from build123d import *

# Parameters (mm, degrees)
SKETCH1_R           = 8.25
SKETCH1_R_2         = 4.25
SKETCH1_R_3         = 15.25
SKETCH1_R_4         = 11.25
SKETCH1_R_5         = 6.25
BOSS_EXTRUDE2_DEPTH = 10
SKETCH1_5_R         = 11.25
CUT_EXTRUDE5_DEPTH  = 7


with BuildPart() as part:
    # Sketch1 → Boss-Extrude2 (new body)
    # profile 1 of 7: a face of its own
    with BuildSketch(Plane.XY):
        with BuildLine():
            Line((64.758616135, -27.860720154), (22.059293714, -16.720850027))
            ThreePointArc((22.059293714, -16.720850027), (26.505216378, -19.659807339), (28.226652646, -24.703650675))
            ThreePointArc((28.226652646, -24.703650675), (20.56881743, -32.932371163), (11.81166092, -25.884925461))
            Line((11.81166092, -25.884925461), (21.633984529, -93.776995906))
            ThreePointArc((21.633984529, -93.776995906), (35.63224039, -76.382762218), (51.976848021, -91.593427362))
            ThreePointArc((51.976848021, -91.593427362), (47.525288564, -102.361722577), (36.769479911, -106.843367773))
            Line((36.769479911, -106.843367773), (86.769284535, -106.703591085))
            ThreePointArc((86.769284535, -106.703591085), (73.507639588, -83.849691589), (99.930570224, -83.823509091))
            Line((99.930570224, -83.823509091), (69.819078019, -31.715739289))
            ThreePointArc((69.819078019, -31.715739289), (70.644447296, -33.706712359), (70.925975067, -35.843520802))
            ThreePointArc((70.925975067, -35.843520802), (56.147411334, -40.887364137), (64.758616135, -27.860720154))
        make_face()
    # profile 2 of 7: a face of its own
    with BuildSketch(Plane.XY):
        with Locations((62.675975067, -35.843520802)):
            Circle(SKETCH1_R)
        with Locations((62.675975067, -35.843520802)):
            Circle(SKETCH1_R_2, mode=Mode.SUBTRACT)
    # profile 3 of 7: a face of its own
    with BuildSketch(Plane.XY):
        with Locations((36.726848021, -91.593427362)):
            Circle(SKETCH1_R_3)
        with Locations((36.726848021, -91.593427362)):
            Circle(SKETCH1_R_4, mode=Mode.SUBTRACT)
    # profile 4 of 7: a face of its own
    with BuildSketch(Plane.XY):
        with Locations((86.726652646, -91.453650675)):
            Circle(SKETCH1_R_3)
        with Locations((86.726652646, -91.453650675)):
            Circle(SKETCH1_R_4, mode=Mode.SUBTRACT)
    # profile 5 of 7: a face of its own
    with BuildSketch(Plane.XY):
        with Locations((19.976652646, -24.703650675)):
            Circle(SKETCH1_R)
        with Locations((19.976652646, -24.703650675)):
            Circle(SKETCH1_R_2, mode=Mode.SUBTRACT)
    # profile 6 of 7: a face of its own
    with BuildSketch(Plane.XY):
        with Locations((36.726848021, -91.593427362)):
            Circle(SKETCH1_R_4)
        with Locations((36.726848021, -91.593427362)):
            Circle(SKETCH1_R_5, mode=Mode.SUBTRACT)
    # profile 7 of 7: a face of its own
    with BuildSketch(Plane.XY):
        with Locations((86.726652646, -91.453650675)):
            Circle(SKETCH1_R_4)
        with Locations((86.726652646, -91.453650675)):
            Circle(SKETCH1_R_5, mode=Mode.SUBTRACT)
    extrude(amount=BOSS_EXTRUDE2_DEPTH)

    # Sketch1<5> → Cut-Extrude5 (cut)
    with BuildSketch(Plane.XY):
        with Locations((86.726652646, -91.453650675)):
            Circle(SKETCH1_5_R)
        with Locations((36.726848021, -91.593427362)):
            Circle(SKETCH1_5_R)
    extrude(amount=CUT_EXTRUDE5_DEPTH, mode=Mode.SUBTRACT)


solid = part.part
Geometry check sheet. Reference: the model listing, model coordinates, mm. A direction names the side the tool comes from. Give positions to 0.01 mm unless a question says otherwise; leave off trailing zeros. Write each loop counter-clockwise with the first axis right and the second up, starting at its lowest first coordinate (ties: lowest second). Pieces come first, ordered by that corner, then holes. Notation, with made-up numbers: (-1.75, 11) - (22.25, 11) arc R19 ccw to (22.25, 40) - close; hole circle Ø4 at (65.25, 80.5). An arc over 180 degrees is marked (long way). Put each result on its own line as item: value.
1. Sectioned sample at C-C, the plane z = 1.25. Enter the section's corners in (x, y).
Ans:
outline: (11.81, -25.88) - (21.63, -93.78) arc R15.25 ccw to (36.77, -106.84) - (86.77, -106.7) arc R15.25 ccw to (99.93, -83.82) - (69.82, -31.72) arc R8.25 ccw to (64.76, -27.86) - (22.06, -16.72) arc R8.25 ccw to start; hole circle Ø8.5 at (19.98, -24.7); hole circle Ø22.5 at (36.73, -91.59); hole circle Ø8.5 at (62.68, -35.84); hole circle Ø22.5 at (86.73, -91.45)
2. Sectioned sample at B-B, the plane x = 89. Enter the section's corners in (y, z), plus the area to 3 significant figures.
Ans:
outline: (-106.53, 0) - (-102.47, 0) - (-102.47, 7) - (-97.28, 7) - (-97.28, 10) - (-106.53, 10) - close; (-85.63, 7) - (-80.44, 7) - (-80.44, 0) - (-64.91, 0) - (-64.91, 10) - (-85.63, 10) - close
area: 227 mm²
3. Thickness scan on line 1 (X direction, y = -94.5, z = 7.25); line 2 (Z direction, x = 40.5, y = -82); line 3 (X direction, y = -90, z = 6). Record the ranges inside material, lowest first.
Ans:
line 1: x = 21.76 to 31.19, 42.26 to 81.27, 92.18 to 101.67
line 2: z = 7 to 10
line 3: x = 21.09 to 25.59, 47.86 to 75.57, 97.88 to 101.91
4. Sectioned sample at A-A, the plane y = -33.5. Enter the section's corners in (x, z), plus the area to 3 significant figures.
Ans:
outline: (12.91, 0) - (59.13, 0) - (59.13, 10) - (12.91, 10) - close; (66.22, 0) - (70.85, 0) - (70.85, 10) - (66.22, 10) - close
area: 508 mm²
5. Set-up check for faces 5 (the cylindrical face through (67.7, -29.3, 4.9)), 6 (the cylindrical face through (34.288, -102.576, 3.451)): record each of +Z, -Z, +X, -X, +Y, -Y from which the full face is reachable in a straight line by a thin tool's end or side.
Ans:
face 5: +Z, -Z, +X, +Y
face 6: -Z
6. Go/stop test with flat-tipped pins: pin 1 (1 mm diameter, centred on x = 56, y = -67.5, fed in from -Z); pin 2 (3 mm diameter, centred on y = -47.5, z = 4, fed in from -X); pin 3 (14.5 mm diameter, centred on x = 86.73, y = -91.45, fed in from -Z); pin 4 (1 mm diameter, centred on y = -70.5, z = 5.5, fed in from +X). Record where each tip stops, or that it passes through.
Ans:
pin 1: stops at z = 0
pin 2: stops at x = 14.72
pin 3: stops at z = 7
pin 4: stops at x = 92.52
7. Sectioned sample at D-D, the plane x = 28.5. Enter the section's corners in (y, z).
Ans:
outline: (-104.43, 0) - (-99.27, 0) - (-99.27, 7) - (-83.92, 7) - (-83.92, 0) - (-18.4, 0) - (-18.4, 10) - (-104.43, 10) - close
8. Draft check along X on faces 1 (the flat face through (92, -96, 7)), 2 (the flat face through (42, -96, 7)), 3 (the flat face through (16.654, -59.356, 4.93)), 4 (the cylindrical face through (99.833, -99.25, 4.93)). Enter one of: +X half, -X half, draft (parallel to the pull), parting line (faces both ways), or undercut.
Ans:
face 1: undercut
face 2: undercut
face 3: -X half
face 4: +X half
